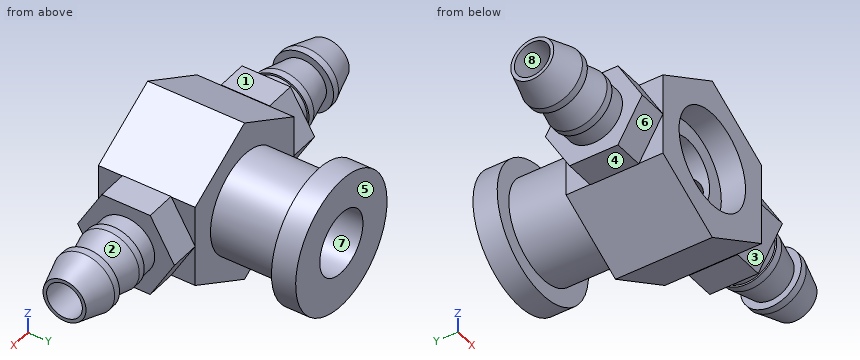
```python
from build123d import *

# Parameters (mm, degrees)
SKETCH1_R            = 5.5
SKETCH1_R_2          = 4.1
BOSS_EXTRUDE1_DEPTH  = 2
SKETCH2_R            = 4.1
BOSS_EXTRUDE2_DEPTH  = 8
SKETCH4_R            = 2.6
BOSS_EXTRUDE3_DEPTH  = 22
BOSS_EXTRUDE4_DEPTH  = 8
BOSS_EXTRUDE5_DEPTH  = 2.5
BOSS_EXTRUDE6_DEPTH  = 2.5
SKETCH8_R            = 2.6
CUT_EXTRUDE1_DEPTH   = 16
SKETCH9_R            = 2.37037037
BOSS_EXTRUDE7_DEPTH  = 1.481481481
SKETCH10_R           = 2.37037037
BOSS_EXTRUDE8_DEPTH  = 1.481481481
SKETCH11_R           = 2.518518519
BOSS_EXTRUDE9_DEPTH  = 0.592592593
SKETCH13_R           = 2.518518519
SKETCH12_R           = 1.925925926
SKETCH14_R           = 2.51851852
BOSS_EXTRUDE10_DEPTH = 0.592592593
SKETCH16_R           = 2.51851852
SKETCH15_R           = 1.77777778
SKETCH17_R           = 1.47777778
CUT_EXTRUDE2_DEPTH   = 31.691734637
SKETCH18_R           = 2.6
CUT_EXTRUDE3_DEPTH   = 6
SKETCH21_R           = 4
CUT_EXTRUDE4_DEPTH   = 2


with BuildPart() as part:
    # Sketch1 → Boss-Extrude1 (new body)
    with BuildSketch(Plane(origin=(0, 0, 0), x_dir=(1, 0, 0), z_dir=(0, 1, 0))):
        with Locations(Location((0, 0, 0), (0, 0, 270))):
            Circle(SKETCH1_R)
        with Locations(Location((0, 0, 0), (0, 0, 270))):
            Circle(SKETCH1_R_2, mode=Mode.SUBTRACT)
    extrude(amount=BOSS_EXTRUDE1_DEPTH)



with BuildPart() as body_2:
    # Sketch2 → Boss-Extrude2 (new body)
    with BuildSketch(Plane(origin=(0, 2, 0), x_dir=(1, 0, 0), z_dir=(0, 1, 0))):
        with Locations(Location((0, 0, 0), (0, 0, 270))):
            Circle(SKETCH2_R)
    extrude(amount=-BOSS_EXTRUDE2_DEPTH)


with BuildPart() as part_1:
    add(part.part)

    add(body_2.part)  # Boss-Extrude3 merges body 2
    # Sketch4 → Boss-Extrude3 (add)
    with BuildSketch(Plane(origin=(0, 2, 0), x_dir=(1, 0, 0), z_dir=(0, 1, 0))):
        with Locations(Location((0, 0, 0), (0, 0, 270))):
            Circle(SKETCH4_R)
    extrude(amount=-BOSS_EXTRUDE3_DEPTH)

    # Sketch5 → Boss-Extrude4 (add)
    with BuildSketch(Plane.XZ.offset(6)):
        Polygon((5.938459912, -3.428571429), (5.938459912, 3.428571429), (0, 6.857142857), (-5.938459912, 3.428571429), (-5.938459912, -3.428571429), (0, -6.857142857), align=None)
    extrude(amount=BOSS_EXTRUDE4_DEPTH)

    # Sketch6 → Boss-Extrude5 (add)
    with BuildSketch(Plane(origin=(5.938459912, 0, 0), x_dir=(0, 0, -1), z_dir=(1, 0, 0))):
        Polygon((0, -14), (3.464101615, -12), (3.464101615, -8), (0, -6), (-3.464101615, -8), (-3.464101615, -12), align=None)
    extrude(amount=BOSS_EXTRUDE5_DEPTH)

    # Sketch7 → Boss-Extrude6 (add)
    with BuildSketch(Plane.ZY.offset(5.938459912)):
        Polygon((0, -14), (3.464101615, -12), (3.464101615, -8), (0, -6), (-3.464101615, -8), (-3.464101615, -12), align=None)
    extrude(amount=BOSS_EXTRUDE6_DEPTH)

    # Sketch8 → Cut-Extrude1 (cut)
    with BuildSketch(Plane(origin=(0, 2, 0), x_dir=(1, 0, 0), z_dir=(0, 1, 0))):
        with Locations(Location((0, 0, 0), (0, 0, 270))):
            Circle(SKETCH8_R)
    extrude(amount=-CUT_EXTRUDE1_DEPTH, mode=Mode.SUBTRACT)


with BuildPart() as cut_extrude1_piece_1:
    # of the separate pieces the step leaves, piece 1, a body of its own (cut_extrude1_pieces)
    add(part_1.part.solids().sort_by_distance((0, 2, 5.5))[0])

    # Sketch9 → Boss-Extrude7 (add)
    with BuildSketch(Plane(origin=(8.438459912, 0, 0), x_dir=(0, 0, -1), z_dir=(1, 0, 0))):
        with Locations((-0.017765093, -10)):
            Circle(SKETCH9_R)
    extrude(amount=BOSS_EXTRUDE7_DEPTH)

    # Sketch10 → Boss-Extrude8 (add)
    with BuildSketch(Plane.ZY.offset(8.438459912)):
        with Locations((0, -10)):
            Circle(SKETCH10_R)
    extrude(amount=BOSS_EXTRUDE8_DEPTH)

    # Sketch11 → Boss-Extrude9 (add)
    with BuildSketch(Plane(origin=(9.919941393, 0, 0), x_dir=(0, 0, -1), z_dir=(1, 0, 0))):
        with Locations((-0.017765093, -10)):
            Circle(SKETCH11_R)
    boss_extrude9 = extrude(amount=BOSS_EXTRUDE9_DEPTH)

    # Sketch13 → Loft1 section 0
    with BuildSketch(Plane(origin=(10.512533986, 0, 0), x_dir=(0, 0, -1), z_dir=(1, 0, 0))):
        with Locations((-0.017765093, -10)):
            Circle(SKETCH13_R)
    # Sketch12 → Loft1 section 1
    with BuildSketch(Plane(origin=(12.882904356, 0, 0), x_dir=(0, 0, -1), z_dir=(1, 0, 0))):
        with Locations((-0.017765093, -10)):
            Circle(SKETCH12_R)
    loft1 = loft()

    # Sketch14 → Boss-Extrude10 (add)
    with BuildSketch(Plane(origin=(12.882904356, 0, 0), x_dir=(0, 0, -1), z_dir=(1, 0, 0))):
        with Locations(Location((-0.017765093, -10, 0), (0, 0, 180))):
            Circle(SKETCH14_R)
    boss_extrude10 = extrude(amount=BOSS_EXTRUDE10_DEPTH)

    # Sketch16 → Loft2 section 0
    with BuildSketch(Plane(origin=(13.475496948, 0, 0), x_dir=(0, 0, -1), z_dir=(1, 0, 0))):
        with Locations((-0.017765093, -10)):
            Circle(SKETCH16_R)
    # Sketch15 → Loft2 section 1
    with BuildSketch(Plane(origin=(15.845867318, 0, 0), x_dir=(0, 0, -1), z_dir=(1, 0, 0))):
        with Locations((-0.017765093, -10)):
            Circle(SKETCH15_R)
    loft2 = loft()

    # Mirror1: Boss-Extrude9, Loft1, Boss-Extrude10, Loft2 across plane
    add(boss_extrude9.mirror(Plane(origin=(0, 0, 0), x_dir=(0, 0, 1), z_dir=(1, 0, 0))))
    add(loft1.mirror(Plane(origin=(0, 0, 0), x_dir=(0, 0, 1), z_dir=(1, 0, 0))))
    add(boss_extrude10.mirror(Plane(origin=(0, 0, 0), x_dir=(0, 0, 1), z_dir=(1, 0, 0))))
    add(loft2.mirror(Plane(origin=(0, 0, 0), x_dir=(0, 0, 1), z_dir=(1, 0, 0))))

    # Sketch17 → Cut-Extrude2 (cut)
    with BuildSketch(Plane(origin=(15.845867318, 0, 0), x_dir=(0, 0, -1), z_dir=(1, 0, 0))):
        with Locations((-0.017765093, -10)):
            Circle(SKETCH17_R)
    extrude(amount=-CUT_EXTRUDE2_DEPTH, mode=Mode.SUBTRACT)

    # Sketch21 → Cut-Extrude4 (cut)
    with BuildSketch(Plane.XZ.offset(14)):
        with Locations(Location((0, 0, 0), (0, 0, 270))):
            Circle(SKETCH21_R)
    extrude(amount=-CUT_EXTRUDE4_DEPTH, mode=Mode.SUBTRACT)


with BuildPart() as cut_extrude1_piece_2:
    # of the separate pieces the step leaves, piece 2, a body of its own (cut_extrude1_pieces)
    add(part_1.part.solids().sort_by_distance((0, -20, 2.6))[0])

    # Sketch18 → Cut-Extrude3 (cut)
    with BuildSketch(Plane.XZ.offset(20)):
        with Locations(Location((0, 0, 0), (0, 0, 90))):
            Circle(SKETCH18_R)
    extrude(amount=-CUT_EXTRUDE3_DEPTH, mode=Mode.SUBTRACT)


solid = cut_extrude1_piece_1.part
```
Verification items for the finished model (mm, model axes). Face numbers are marked on the shaded views. A direction names the side the tool comes from. Coordinates: 2 decimals unless noted, no trailing zeros. Loops run counter-clockwise (first coordinate to the right, second up) from the corner with the lowest first, then second, coordinate; pieces in that order, holes last. Notation, with made-up numbers: (82, 74.5) - (90, 74.5) arc R17 ccw to (90, 101.5) - close; hole circle Ø4 at (67, 15.5). An arc over 180 degrees is marked (long way). Answer as a JSON object with one key per item and string values.
(1) Cross-section at B-B, the plane x = 6.5. Record the boundary of the cut face in (y, z), then the cut area to 3 significant figures.
Response:
{"outline": "(-14, 0) - (-12, -3.46) - (-8, -3.46) - (-6, 0) - (-8, 3.46) - (-12, 3.46) - close; hole circle Ø2.96 at (-10, 0.02)", "area": "34.7 mm²"}
(2) Cross-section at D-D, the plane x = -9. Record the boundary of the cut face in (y, z).
Response:
{"outline": "circle Ø4.74 at (-10, 0); hole circle Ø2.96 at (-10, 0.02)"}
(3) Mould release check, pull along Z, two halves, no side actions. Record for the marked faces 5, 6, 7 and 8: pulls with the +Z half, pulls with the -Z half, needs draft (parallel to the pull), parting line crosses it, or undercut.
Response:
{"face 5": "needs draft", "face 6": "pulls with the -Z half", "face 7": "undercut", "face 8": "undercut"}
(4) Cross-section at A-A, the plane z = 4.75. Record the boundary of the cut face in (x, y), then the cut area to 3 significant figures.
Response:
{"outline": "(-3.65, -14) - (3.65, -14) - (3.65, -6) - (-3.65, -6) - close; (-2.77, 0) - (2.77, 0) - (2.77, 2) - (-2.77, 2) - close", "area": "69.5 mm²"}
(5) Access from +Z, -Z, +X, -X, +Y, -Y to the whole of each face (thin tool, end or side, straight path). Record for the marked faces 1, 2, 3 and 4.
Response:
{"face 1": "+Z, -X, +Y, -Y", "face 2": "none", "face 3": "-Z, +X, -Y", "face 4": "-Z, -X, +Y, -Y"}
(6) Scan lines: line 1 along X through (y, z) = (-12.9, 0); line 2 along X through (y, z) = (-2.5, 0); line 3 along Y through (x, z) = (13, 0). Record each from-to range of solid material in increasing order.
Response:
{"line 1": "x = -8.44 to -4, 4 to 8.44", "line 2": "x = -4.1 to -2.6, 2.6 to 4.1", "line 3": "y = -12.52 to -11.48, -8.52 to -7.48"}
(7) Go/stop test with flat-tipped pins: pin 1 Ø2.5 at (x, y) = (7.5, -10) entering from -Z; pin 2 Ø2 at (x, y) = (-6.5, -10.5) entering from -Z; pin 3 Ø1.2 at (x, y) = (7.5, -10.5) entering from +Z; pin 4 Ø1.8 at (y, z) = (-10, 0.02) entering from -X. Record where each tip stops, or that it passes through.
Response:
{"pin 1": "stops at z = -3.46", "pin 2": "stops at z = -3.68", "pin 3": "stops at z = 3.46", "pin 4": "passes through"}
(8) Cross-section at C-C, the plane y = 0.5. Record the boundary of the cut face in (x, z), then the cut area to 3 significant figures.
Response:
{"outline": "circle Ø11 at (0, 0); hole circle Ø5.2 at (0, 0)", "area": "73.8 mm²"}
